The listing builds one solid part. Answer for the finished solid, in the listing's coordinates (mm). A direction names the side the tool comes from. Give positions to 0.01 mm unless a question says otherwise; leave off trailing zeros. Write each loop counter-clockwise with the first axis right and the second up, starting at its lowest first coordinate (ties: lowest second). Pieces come first, ordered by that corner, then holes. Notation, with made-up numbers: (61.25, 10.25) - (94.25, 10.25) arc R18 cw to (94.25, 41.25) - close; hole circle Ø9 at (25, 38.25). An arc over 180 degrees is marked (long way). One line per item, written item: value. Start each with the question number.
from build123d import *

# Parameters (mm, degrees)
SKETCH1_W           = 35
SKETCH1_H           = 25
BOSS_EXTRUDE1_DEPTH = 20
SKETCH5_W           = 1.5
SKETCH5_H           = 6
BOSS_EXTRUDE2_DEPTH = 35
SKETCH2_R           = 4.5
CUT_EXTRUDE1_DEPTH  = 21
SKETCH3_R           = 2.5
CUT_EXTRUDE4_DEPTH  = 27.5
SKETCH4_R           = 5
SKETCH4_R_2         = 2.5
CUT_EXTRUDE5_DEPTH  = 5


with BuildPart() as part:
    # Sketch1 → Boss-Extrude1 (new body)
    with BuildSketch(Plane(origin=(0, 0, 0), x_dir=(1, 0, 0), z_dir=(0, 1, 0))):
        with Locations((17.5, 12.5)):
            Rectangle(SKETCH1_W, SKETCH1_H)
    extrude(amount=BOSS_EXTRUDE1_DEPTH)

    # Sketch5 → Boss-Extrude2 (add, through all)
    with BuildSketch(Plane(origin=(35, 0, 0), x_dir=(0, 0, -1), z_dir=(1, 0, 0))):
        with Locations((-0.75, 10)):
            Rectangle(SKETCH5_W, SKETCH5_H)
    extrude(amount=-BOSS_EXTRUDE2_DEPTH)

    # Sketch2 → Cut-Extrude1 (cut, through all)
    with BuildSketch(Plane(origin=(0, 20, 0), x_dir=(1, 0, 0), z_dir=(0, 1, 0))):
        with Locations((17.5, 14.5)):
            Circle(SKETCH2_R)
    extrude(amount=-CUT_EXTRUDE1_DEPTH, mode=Mode.SUBTRACT)

    # Sketch3 → Cut-Extrude4 (cut, through all)
    with BuildSketch(Plane(origin=(0, 0, -25), x_dir=(-1, 0, 0), z_dir=(0, 0, -1))):
        with Locations((-7.5, 10)):
            Circle(SKETCH3_R)
        with Locations((-27.5, 10)):
            Circle(SKETCH3_R)
    extrude(amount=-CUT_EXTRUDE4_DEPTH, mode=Mode.SUBTRACT)

    # Sketch4 → Cut-Extrude5 (cut)
    with BuildSketch(Plane(origin=(0, 0, -25), x_dir=(-1, 0, 0), z_dir=(0, 0, -1))):
        with Locations((-7.5, 10)):
            Circle(SKETCH4_R)
        with Locations((-7.5, 10)):
            Circle(SKETCH4_R_2, mode=Mode.SUBTRACT)
        with Locations((-27.5, 10)):
            Circle(SKETCH4_R)
        with Locations((-27.5, 10)):
            Circle(SKETCH4_R_2, mode=Mode.SUBTRACT)
    extrude(amount=-CUT_EXTRUDE5_DEPTH, mode=Mode.SUBTRACT)


solid = part.part
Item 1: Find section D-D on y = 14.25. Determine the outline of the cut face in (x, z), plus the area to 3 significant figures.
Item 2: Find section B-B on x = 17.5. Determine the outline of the cut face in (y, z).
Item 3: Find section A-A on z = -14.5. Determine the outline of the cut face in (x, y).
Item 4: For faces 5 (the flat face through (17, 3, 0)), 6 (the cylindrical face through (31.185, 13.379, -22.535)), 7 (the flat face through (17, 16, 0)), determine the directions among +Z, -Z, +X, -X, +Y, -Y from which every point of the face is accessible in a straight line to the end or side of a thin tool.
Item 5: Each of these flat-tipped pins is pushed along its axis until it touches: pin 1 Ø5 at (x, y) = (7, 12) entering from -Z; pin 2 Ø1 at (x, y) = (10, 15.5) entering from +Z; pin 3 Ø1.6 at (x, z) = (18, 1) entering from +Y. Where does it stop, or does it pass through?
Item 6: The mould has two halves that part along Y. Classify faces 1 (the flat face through (17, 10, -25)), 2 (the flat face through (18, 13, 1)), 3 (the cylindrical face through (2.73, 11.5, -22.54)), 4 (the cylindrical face through (8.04, 7.56, -9.4)): +Y half, -Y half, draft (parallel to the pull), parting line (faces both ways), or undercut.
Item 7: Straight lines are drawn through the part: line 1 along X through (y, z) = (6.5, -14.5); line 2 along X through (y, z) = (8.5, -0.5); line 3 along Y through (x, z) = (27.5, -11.75). For each, find the intervals that lie inside material, in ascending order.
Item 8: Find section C-C on y = 10. Determine the outline of the cut face in (x, z).
Values:
1. outline: (0, -25) - (4.87, -25) - (4.87, -20) - (10.13, -20) - (10.13, -25) - (24.87, -25) - (24.87, -20) - (30.13, -20) - (30.13, -25) - (35, -25) - (35, 0) - (0, 0) - close; hole circle Ø9 at (17.5, -14.5)
1. area: 759 mm^2
2. outline: (0, -25) - (20, -25) - (20, -19) - (0, -19) - close; (0, -10) - (20, -10) - (20, 0) - (13, 0) - (13, 1.5) - (7, 1.5) - (7, 0) - (0, 0) - close
3. outline: (0, 0) - (13, 0) - (13, 20) - (0, 20) - close; (22, 0) - (35, 0) - (35, 20) - (22, 20) - close; hole circle Ø5 at (7.5, 10); hole circle Ø5 at (27.5, 10)
4. face 5: +Z, +X, -X, -Y
4. face 6: -Z
4. face 7: +Z, +X, -X, +Y
5. pin 1: z = -20
5. pin 2: z = 0
5. pin 3: y = 13
6. face 1: draft
6. face 2: +Y half
6. face 3: undercut
6. face 4: undercut
7. line 1: 0 to 13, 22 to 35
7. line 2: 0 to 5.5, 9.5 to 25.5, 29.5 to 35
7. line 3: 0 to 7.5, 12.5 to 20
8. outline: (0, -25) - (2.5, -25) - (2.5, -20) - (5, -20) - (5, 1.5) - (0, 1.5) - close; (10, -20) - (12.5, -20) - (12.5, -25) - (22.5, -25) - (22.5, -20) - (25, -20) - (25, 1.5) - (10, 1.5) - close; (30, -20) - (32.5, -20) - (32.5, -25) - (35, -25) - (35, 1.5) - (30, 1.5) - close; hole circle Ø9 at (17.5, -14.5)
